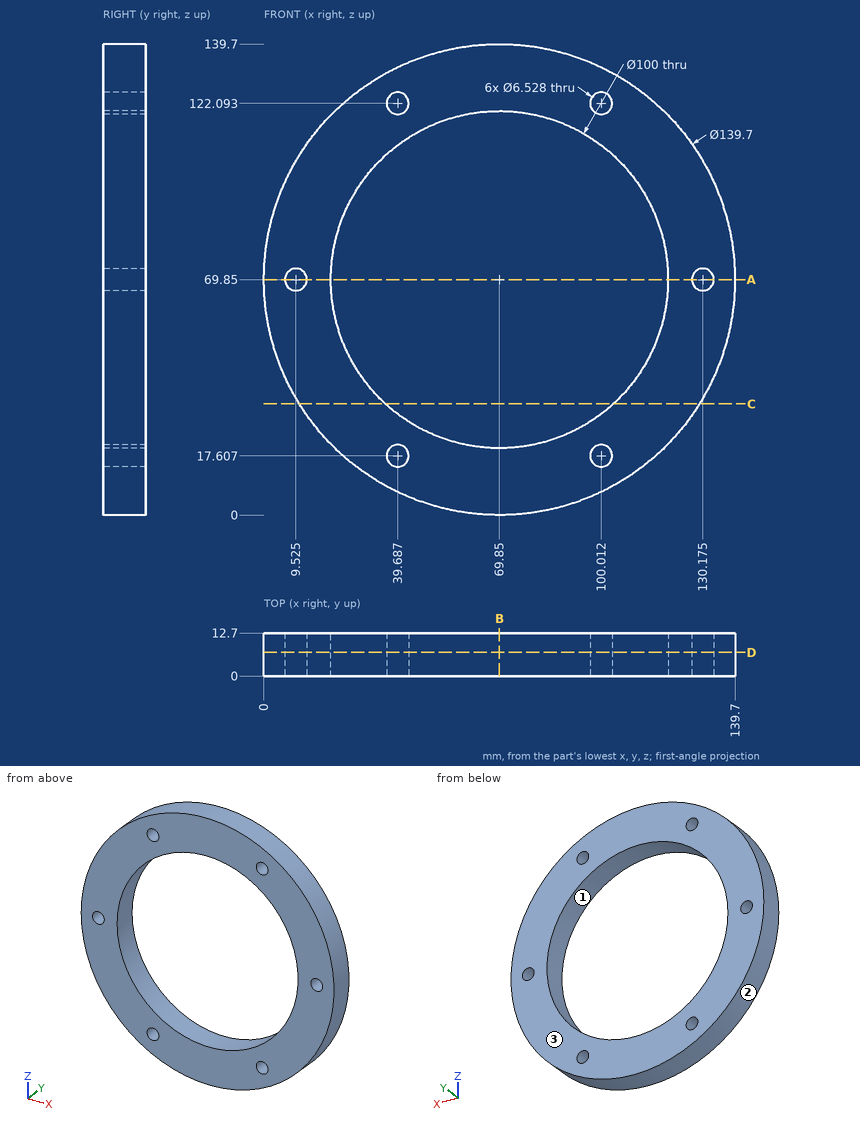
For this review, use the dimensioned drawing (mm, ordinates from the lowest corner) and the shaded views. Round coordinates to 2 decimals unless told otherwise and drop trailing zeros. Order: outer loops, then holes, each group sorted by start corner. A loop starts at its lowest first (then second) coordinate and runs counter-clockwise, first axis right, second up. Notation, with made-up numbers: (12.25, -7) -> (36.25, -7) arc R14 cw to (36.25, 4) -> close; hole circle Ø10 at (72.25, 0). An arc over 180 degrees is marked (long way). One line per item, written item: value. Start each with the question number.
Q1. Take a section at D-D (y = 7). Count the separate pieces of the cut face and the enclosed holes in it, and give its area (3 significant figures).
Q2. Mouldability with a two-part tool opening along X and no side actions: class the marked faces 1, 2 and 3 as released by +X, released by -X, zero draft, split by the parting line, or undercut.
Q3. Take a section at A-A (z = 69.85). Write out the cut boundary in (x, y).
Q4. Take a section at B-B (x = 69.85). Write out the cut boundary in (y, z), and give its area (3 significant figures).
Q5. Wall thickness on line 1 (Z direction, x = 99.5, y = 8.75) (1 decimal); line 2 (X direction, y = 7.75, z = 106) (1 decimal); line 3 (X direction, y = 8.75, z = 97.5) (1 decimal): over which ranges is each line inside the solid? List them lowest first.
Q6. Clearance check with flat-ended pins moving along their axes: pin 1 Ø6 at (x, y) = (80.5, 10.5) entering from -Z; pin 2 Ø5 at (y, z) = (10, 15) entering from -X (1 decimal); pin 3 Ø2 at (x, y) = (104, 9) entering from -Z. State where each tip first meets the part, or that it passes through.
Q7. Take a section at C-C (z = 33). Write out the cut boundary in (x, y) (1 decimal), and give its area (3 significant figures).
Reported:
1. separate pieces: 1
1. enclosed holes: 7
1. area: 7,270 mm2
2. face 1: undercut
2. face 2: split by the parting line
2. face 3: zero draft
3. outline: (0, 0) -> (6.26, 0) -> (6.26, 12.7) -> (0, 12.7) -> close; (12.79, 0) -> (19.85, 0) -> (19.85, 12.7) -> (12.79, 12.7) -> close; (119.85, 0) -> (126.91, 0) -> (126.91, 12.7) -> (119.85, 12.7) -> close; (133.44, 0) -> (139.7, 0) -> (139.7, 12.7) -> (133.44, 12.7) -> close
4. outline: (0, 0) -> (12.7, 0) -> (12.7, 19.85) -> (0, 19.85) -> close; (0, 119.85) -> (12.7, 119.85) -> (12.7, 139.7) -> (0, 139.7) -> close
4. area: 504 mm2
5. line 1: z = 6.6 to 14.4, 20.8 to 29.6, 110.1 to 118.9, 125.3 to 133.1
5. line 2: x = 10.1 to 35.3, 104.4 to 129.6
5. line 3: x = 5.7 to 28.2, 111.5 to 134
6. pin 1: stops at z = 0.42
6. pin 2: stops at x = 23.6
6. pin 3: stops at z = 8.37
7. outline: (10.5, 0) -> (36.1, 0) -> (36.1, 12.7) -> (10.5, 12.7) -> close; (103.6, 0) -> (129.2, 0) -> (129.2, 12.7) -> (103.6, 12.7) -> close
7. area: 649 mm2
